from build123d import *

# Parameters (mm, degrees)
SKETCH1_W               = 80
SKETCH1_H               = 70
BOSS_EXTRUDE1_DEPTH     = 8
FILLET1_R               = 5
CUT_EXTRUDE1_DEPTH      = 54.749418602
CUT_EXTRUDE1_DEPTH_BACK = 18
SKETCH2_R               = 2.25
CUT_EXTRUDE2_DEPTH      = 54.749418602
CUT_EXTRUDE2_DEPTH_BACK = 1
SKETCH2_3_R             = 1.25
SKETCH2_3_W             = 5
SKETCH2_3_H             = 11.5
SKETCH3_R               = 2.5
CUT_EXTRUDE3_DEPTH      = 31


with BuildPart() as part:
    # Sketch1 → Boss-Extrude1 (new body)
    with BuildSketch(Plane(origin=(0, 0, 0), x_dir=(1, 0, 0), z_dir=(0, 1, 0))):
        Rectangle(SKETCH1_W, SKETCH1_H)
    extrude(amount=BOSS_EXTRUDE1_DEPTH)

    # Fillet1
    fillet1_edges = [part.edges().sort_by_distance(p)[0] for p in [
        (40, 4, 35),
        (-40, 4, 35),
        (-40, 4, -35),
        (40, 4, -35),
    ]]
    fillet(fillet1_edges, radius=FILLET1_R)

    # Sketch2 → Cut-Extrude1 (cut, two sides: drawn at the far end of the back side and taken through both)
    # profile 1 of 5: a face of its own
    with BuildSketch(Plane(origin=(0, 8, 0), x_dir=(1, 0, 0), z_dir=(0, 1, 0)).offset(-CUT_EXTRUDE1_DEPTH_BACK)):
        with BuildLine():
            Line((-11.034039005, -5.017602297), (5.415960995, -5.017602297))
            ThreePointArc((5.415960995, -5.017602297), (2.111359022, -3.973142202), (0.007287445, -1.219204313))
            ThreePointArc((0.007287445, -1.219204313), (-2.623258806, 0.732397703), (0.007287445, 2.683999719))
            ThreePointArc((0.007287445, 2.683999719), (2.111359022, 5.437937608), (5.415960995, 6.482397703))
            Line((5.415960995, 6.482397703), (-11.034039005, 6.482397703))
            Line((-11.034039005, 6.482397703), (-11.034039005, -5.017602297))
        make_face()
    # profile 2 of 5: a face of its own
    with BuildSketch(Plane(origin=(0, 8, 0), x_dir=(1, 0, 0), z_dir=(0, 1, 0)).offset(-CUT_EXTRUDE1_DEPTH_BACK)):
        with BuildLine():
            ThreePointArc((0.007287445, -1.219204313), (11.165960995, 0.732397703), (0.007287445, 2.683999719))
            ThreePointArc((0.007287445, 2.683999719), (-2.623258806, 0.732397703), (0.007287445, -1.219204313))
        make_face()
        with Locations((5.415960995, 0.732397703)):
            Circle(SKETCH2_R, mode=Mode.SUBTRACT)
    # profile 3 of 5: a face of its own
    with BuildSketch(Plane(origin=(0, 8, 0), x_dir=(1, 0, 0), z_dir=(0, 1, 0)).offset(-CUT_EXTRUDE1_DEPTH_BACK)):
        with Locations((5.415960995, 0.732397703)):
            Circle(SKETCH2_R)
    # profile 4 of 5: a face of its own
    with BuildSketch(Plane(origin=(0, 8, 0), x_dir=(1, 0, 0), z_dir=(0, 1, 0)).offset(-CUT_EXTRUDE1_DEPTH_BACK)):
        with BuildLine():
            ThreePointArc((5.415960995, 6.482397703), (9.481824987, 4.798261695), (11.165960995, 0.732397703))
            Line((11.165960995, 0.732397703), (11.165960995, 6.482397703))
            Line((11.165960995, 6.482397703), (5.415960995, 6.482397703))
        make_face()
    # profile 5 of 5: a face of its own
    with BuildSketch(Plane(origin=(0, 8, 0), x_dir=(1, 0, 0), z_dir=(0, 1, 0)).offset(-CUT_EXTRUDE1_DEPTH_BACK)):
        with BuildLine():
            Line((11.165960995, -5.017602297), (11.165960995, 0.732397703))
            ThreePointArc((11.165960995, 0.732397703), (9.481824987, -3.333466289), (5.415960995, -5.017602297))
            Line((5.415960995, -5.017602297), (11.165960995, -5.017602297))
        make_face()
    extrude(amount=CUT_EXTRUDE1_DEPTH + CUT_EXTRUDE1_DEPTH_BACK, mode=Mode.SUBTRACT)

    # Sketch2_3 → Cut-Extrude2 (cut, two sides: drawn at the far end of the back side and taken through both)
    # profile 1 of 4: a face of its own
    with BuildSketch(Plane(origin=(0, 8, 0), x_dir=(1, 0, 0), z_dir=(0, 1, 0)).offset(-CUT_EXTRUDE2_DEPTH_BACK)):
        Polygon((11.165960995, 6.482397703), (11.165960995, 0.732397703), (11.165960995, -5.017602297), (16.165960995, -5.017602297), (16.165960995, 6.482397703), align=None)
        with Locations((14.165960995, 0.732397703)):
            Circle(SKETCH2_3_R, mode=Mode.SUBTRACT)
    # profile 2 of 4: a face of its own
    with BuildSketch(Plane(origin=(0, 8, 0), x_dir=(1, 0, 0), z_dir=(0, 1, 0)).offset(-CUT_EXTRUDE2_DEPTH_BACK)):
        with Locations((14.165960995, 0.732397703)):
            Circle(SKETCH2_3_R)
    # profile 3 of 4: a face of its own
    with BuildSketch(Plane(origin=(0, 8, 0), x_dir=(1, 0, 0), z_dir=(0, 1, 0)).offset(-CUT_EXTRUDE2_DEPTH_BACK)):
        with Locations((-13.534039005, 0.732397703)):
            Rectangle(SKETCH2_3_W, SKETCH2_3_H)
        with Locations((-14.034039005, 0.732397703)):
            Circle(SKETCH2_3_R, mode=Mode.SUBTRACT)
    # profile 4 of 4: a face of its own
    with BuildSketch(Plane(origin=(0, 8, 0), x_dir=(1, 0, 0), z_dir=(0, 1, 0)).offset(-CUT_EXTRUDE2_DEPTH_BACK)):
        with Locations((-14.034039005, 0.732397703)):
            Circle(SKETCH2_3_R)
    extrude(amount=CUT_EXTRUDE2_DEPTH + CUT_EXTRUDE2_DEPTH_BACK, mode=Mode.SUBTRACT)

    # Sketch3 → Cut-Extrude3 (cut)
    with BuildSketch(Plane(origin=(0, 8, 0), x_dir=(1, 0, 0), z_dir=(0, 1, 0))):
        with Locations(Location((28, 23, 0), (0, 0, 270))):
            Circle(SKETCH3_R)
        with Locations(Location((28, -23, 0), (0, 0, 270))):
            Circle(SKETCH3_R)
        with Locations(Location((-28, 23, 0), (0, 0, 270))):
            Circle(SKETCH3_R)
        with Locations(Location((-28, -23, 0), (0, 0, 270))):
            Circle(SKETCH3_R)
    extrude(amount=-CUT_EXTRUDE3_DEPTH, mode=Mode.SUBTRACT)


solid = part.part
Verification items for the finished model (mm, model axes). A direction names the side the tool comes from. Coordinates: 2 decimals unless noted, no trailing zeros. Order: outer loops, then holes, each group sorted by start corner. A loop starts at its lowest first (then second) coordinate and runs counter-clockwise, first axis right, second up.
Item 1: Section check B-B, the plane z = 23. Enter the section's corners in (x, y).
Filled in:
outline: (-40, 0) - (-30.5, 0) - (-30.5, 8) - (-40, 8) - close; (-25.5, 0) - (25.5, 0) - (25.5, 8) - (-25.5, 8) - close; (30.5, 0) - (40, 0) - (40, 8) - (30.5, 8) - close
Item 2: Material ranges on L1, parallel to X at y = 5.5, z = 23; L2, parallel to X at y = 3, z = 3.5; L3, parallel to Z at x = 26.5, y = 6.25, recorded low to high.
Filled in:
L1: x = -40 to -30.5, -25.5 to 25.5, 30.5 to 40
L2: x = -40 to -11.03, 11.17 to 40
L3: z = -35 to -25, -21 to 21, 25 to 35
Item 3: Section check D-D, the plane y = 5.5. Enter the section's corners in (x, z).
Filled in:
outline: (-40, -30) arc R5 ccw to (-35, -35) - (35, -35) arc R5 ccw to (40, -30) - (40, 30) arc R5 ccw to (35, 35) - (-35, 35) arc R5 ccw to (-40, 30) - close; hole circle Ø5 at (-28, -23); hole circle Ø5 at (-28, 23); hole (-11.03, -6.48) - (11.17, -6.48) - (11.17, 5.02) - (-11.03, 5.02) - close; hole circle Ø5 at (28, -23); hole circle Ø5 at (28, 23)
Item 4: Access from +Z, -Z, +X, -X, +Y, -Y to the whole of each face (thin tool, end or side, straight path). Record for faces 1 (the face through (-11.034, 3, -1)), 2 (the face through (0, 4, -35)), 3 (the face through (14, 7, -1)).
Filled in:
face 1: +Y, -Y
face 2: -Z, +X, -X, +Y, -Y
face 3: +Y
Item 5: Section check A-A, the plane z = 3. Enter the section's corners in (x, y).
Filled in:
outline: (-40, 0) - (-11.03, 0) - (-11.03, 7) - (-16.03, 7) - (-16.03, 8) - (-40, 8) - close; (11.17, 0) - (40, 0) - (40, 8) - (16.17, 8) - (16.17, 7) - (11.17, 7) - close
Item 6: Section check C-C, the plane x = -28. Enter the section's corners in (y, z), then the cut area to 3 significant figures.
Filled in:
outline: (0, -35) - (8, -35) - (8, -25.5) - (0, -25.5) - close; (0, -20.5) - (8, -20.5) - (8, 20.5) - (0, 20.5) - close; (0, 25.5) - (8, 25.5) - (8, 35) - (0, 35) - close
area: 480 mm2
Item 7: Release check for a two-part mould opening along Z. For faces 4 (the face through (-26.31, 4.06, -24.84)), 5 (the face through (-39, 4, 33)), 6 (the face through (40, 4, 0)) record: +Z half, -Z half, draft (parallel to the pull), parting line (faces both ways), or undercut.
Filled in:
face 4: undercut
face 5: +Z half
face 6: draft
Item 8: Depth check by flat-ended pin: pin 1 (1.5 mm diameter, centred on x = 14.5, z = 0.5, fed in from +Y). Enter the tip coordinate at first touch or a pass-through.
Filled in:
pin 1: stops at y = 7
